Autodesk Fusion 360 part; units mm, degrees
sketch "Sketch1" plane through (0, 0, 0) normal (1, 0, 0) x (0, 1, 0)
  line L0 (0, 0) -> (100, 0)
  line L1 (100, 0) -> (100, 76) construction
  line L2 (0, 76) -> (0, 0) construction
  line L3 (0, 76) -> (100, 76) construction
  arc A0 (22, 76) -> (0, 54) centre (22, 54) ccw
  arc A1 (100, 54) -> (78, 76) centre (78, 54) ccw
  line L4 (22, 45.5) -> (78, 45.5)
  line L5 (22, 62.5) -> (78, 62.5)
  arc A2 (22, 62.5) -> (22, 45.5) centre (22, 54) ccw
  arc A3 (78, 45.5) -> (78, 62.5) centre (78, 54) ccw
  circle A4 centre (50, 96) radius 7.5
  line L6 (34, 81) -> (34, 96)
  line L7 (66, 81) -> (66, 96)
  arc A5 (29, 76) -> (34, 81) centre (29, 81) ccw
  arc A6 (66, 81) -> (71, 76) centre (71, 81) ccw
  line L8 (0, 0) -> (0, 54)
  line L9 (100, 0) -> (100, 54)
  line L10 (78, 76) -> (22, 76)
  arc A7 (66, 96) -> (34, 96) centre (50, 96) ccw
  line L11 (0, 8) -> (100, 8)
  line L12 (0, 16) -> (100, 16)
  line L13 (100, 28) -> (0, 28)
  dimension "d1" = 100
  dimension "d3" = 76
  dimension "d4" = 44
  dimension "d5" = 44
  dimension "d6" = 17
  dimension "d7" = 22
  dimension "d8" = 17
  dimension "d9" = 78
  dimension "d10" = 54
  dimension "d11" = 54
  dimension "d12" = 15
  dimension "d13" = 32
  dimension "d14" = 50
  dimension "d15" = 50
  dimension "d16" = 96
  dimension "d17" = 96
  dimension "d18" = 10
  dimension "d19" = 10
  dimension "d20" = 8
  dimension "d21" = 16
  dimension "d26" = 28
sketch "Sketch2" plane through (0, 0, 0) normal (0, 0, 1) x (1, 0, 0)
  line L0 (0, 0) -> (0, 81) construction
  circle A0 centre (0, 19) radius 6
  circle A1 centre (0, 81) radius 6
  dimension "d39" = 12
  dimension "d40" = 12
  dimension "d41" = 81
  dimension "d42" = 19
  dimension "d44" = 81
extrude "Extrude1" add sketch "Sketch1" along normal blind 10 from surface at 25 contours A0 A1 L8 L9 L10 L13 | L6 L7 A5 A6 L10 A7 makes body 1
extrude "Extrude2" add sketch "Sketch1" against normal blind 10 from surface at -25 separate body contours A0 A1 L8 L9 L10 L13 makes body 2
extrude "Extrude8" add sketch "Sketch1" along normal up to surface (-35 mm away) and the other way up to surface (-35 mm away) contours L8 L9 L12 L13 bodies 1 2
extrude "Extrude9" add sketch "Sketch1" along normal up to surface (35 mm away) and the other way up to surface (35 mm away) contours L8 L9 L11 L12 bodies 1
extrude "Extrude10" cut sketch "Sketch1" along normal blind 19 and the other way blind 19 contours L8 L9 L11 L12 bodies 1
extrude "Extrude11" add sketch "Sketch1" along normal up to surface (-35 mm away) and the other way up to surface (-35 mm away) contours L0 L8 L9 L11 bodies 1
extrude "Extrude12" cut sketch "Sketch1" along normal blind 9 and the other way blind 9 contours L0 L8 L9 L11 bodies 1
extrude "Extrude13" cut sketch "Sketch2" along normal through all bodies 1
equation "d3 = 54 mm + 22 mm"
equation "d6 = ( 8.5 * 2 ) * 1 mm"
equation "d7 = ( 100 mm / 2 mm ) * 1 mm - ( 56 / 2 ) * 1 mm"
equation "d9 = 100 mm - 22 mm"
equation "d11 = d10"
equation "d16 = d10 + 42 mm"
equation "d17 = d16"
equation "d41 = 100 mm - 19 mm"
equation "d44 = d41"
equation "d45 = 35 mm - 10 mm"
equation "d46 = -35 mm + 10 mm"
Build history of the part. All positions in model axes, mm. A direction names the side the tool comes from. Coordinates: 2 decimals unless noted, no trailing zeros. Order: outer loops, then holes, each group sorted by start corner. A loop starts at its lowest first (then second) coordinate and runs counter-clockwise, first axis right, second up. Notation, with made-up numbers: (-16.75, -33) - (27.25, -33) arc R23 ccw to (27.25, -12) - close; hole circle Ø2 at (11.5, 53). An arc over 180 degrees is marked (long way). Write each question's results on one line, items separated by ' | '. Start each with the question number.
Item 1: Band-saw the part on A-A on y = 50. Write the cut outline in (x, z), and give its area (3 significant figures).
Item 2: Band-saw the part on D-D on z = 70.5. Write the cut outline in (x, y).
Item 3: Tool access for faces 1 (the face through (-29.93, 13.502, 54.187)), 2 (the face through (-25, 49, 42)), 3 (the face through (30, 26, 76)), 4 (the face through (30, 66, 88)), 5 (the face through (-14, 49, 8)): list every direction of +Z, -Z, +X, -X, +Y, -Y with a clear straight run to the whole face (end or side of a thin tool).
Item 4: Wall check: probe 1 along Y at (x, z) = (0, 24.5); probe 2 along X at (y, z) = (79, 62.5); probe 3 along X at (y, z) = (19, 20.5). Give the ranges that are in metal, low to high. Write a range as [from, to].
Item 5: Band-saw the part on C-C on z = 21. Write the cut outline in (x, y), and give its area (3 significant figures).
Item 6: Flat gauge pins, fed straight in: pin 1 (5 mm diameter, centred on x = 29.5, y = 45.5, fed in from +Z); pin 2 (2 mm diameter, centred on x = -25, y = 62.5, fed in from +Z); pin 3 (3 mm diameter, centred on x = 13.5, y = 32, fed in from +Z). Where does each tip first touch, or does it go through?
Item 7: Band-saw the part on B-B on x = -11. Write the cut outline in (y, z), and give its area (3 significant figures).
Item 8: Mould opens along Y. For faces 6 (the face through (29.93, 53.461, 102.654)), 7 (the face through (30, 34, 88)), 8 (the face through (35, 49, 44)) say: released by +Y, released by -Y, zero draft, split by the parting line, or undercut.
Numbers:
1) outline: (-35, 0) - (-9, 0) - (-9, 8) - (-19, 8) - (-19, 16) - (19, 16) - (19, 8) - (9, 8) - (9, 0) - (35, 0) - (35, 45.5) - (25, 45.5) - (25, 28) - (-25, 28) - (-25, 45.5) - (-35, 45.5) - close; (-35, 62.5) - (-25, 62.5) - (-25, 76) - (-35, 76) - close; (25, 62.5) - (35, 62.5) - (35, 88.5) - (25, 88.5) - close; (25, 103.5) - (35, 103.5) - (35, 112) - (25, 112) - close | area: 2,340 mm^2
2) outline: (-35, 7.45) - (-25, 7.45) - (-25, 92.55) - (-35, 92.55) - close; (25, 7.45) - (35, 7.45) - (35, 92.55) - (25, 92.55) - close
3) face 1: +X, -X | face 2: +Z, +Y, -Y | face 3: +Z, +X, -X, -Y | face 4: +Z, +X, -X, +Y | face 5: +Y, -Y
4) probe 1: [0, 13], [25, 75], [87, 100] | probe 2: [-35, -25], [25, 35] | probe 3: [-35, -6], [6, 35]
5) outline: (-35, 0) - (35, 0) - (35, 100) - (-35, 100) - close; hole circle Ø12 at (0, 19); hole circle Ø12 at (0, 81) | area: 6,770 mm^2
6) pin 1: z = 111.87 | pin 2: z = 76 | pin 3: z = 28
7) outline: (0, 0) - (100, 0) - (100, 8) - (0, 8) - close; (0, 16) - (100, 16) - (100, 28) - (0, 28) - close | area: 2,000 mm^2
8) face 6: undercut | face 7: released by -Y | face 8: zero draft
